Design review of the part built by this model. Coordinates are the model's own, in mm. A direction names the side the tool comes from. Coordinates: 2 decimals unless noted, no trailing zeros. Loops run counter-clockwise (first coordinate to the right, second up) from the corner with the lowest first, then second, coordinate; pieces in that order, holes last. Notation, with made-up numbers: (19, 44.25) -> (30, 44.25) arc R31 cw to (30, 73.25) -> close; hole circle Ø1 at (47.25, 49.25). An arc over 180 degrees is marked (long way). Answer in a Markdown table with one row per item.
```python
from build123d import *

# Parameters (mm, degrees)
BOSS_EXTRUDE1_DEPTH                   = 9
BOSS_EXTRUDE1_DEPTH_BACK              = 9
TAP_DRILL_FOR_M4_TAP1_D               = 3.3
TAP_DRILL_FOR_M4_TAP1_DEPTH           = 25
TAP_DRILL_FOR_M4_TAP1_TIP             = 0.991420021
TAP_DRILL_FOR_M4_TAP1_ON_FACE_2_D     = 3.3
TAP_DRILL_FOR_M4_TAP1_ON_FACE_2_DEPTH = 25
TAP_DRILL_FOR_M4_TAP1_ON_FACE_2_TIP   = 0.991420021
TAP_DRILL_FOR_M4_TAP1_ON_FACE_3_D     = 3.3
TAP_DRILL_FOR_M4_TAP1_ON_FACE_3_DEPTH = 25
TAP_DRILL_FOR_M4_TAP1_ON_FACE_3_TIP   = 0.991420021
TAP_DRILL_FOR_M4_TAP1_ON_FACE_4_D     = 3.3
TAP_DRILL_FOR_M4_TAP1_ON_FACE_4_DEPTH = 25
TAP_DRILL_FOR_M4_TAP1_ON_FACE_4_TIP   = 0.991420021
TAP_DRILL_FOR_M4_TAP1_ON_FACE_5_D     = 3.3
TAP_DRILL_FOR_M4_TAP1_ON_FACE_5_DEPTH = 25
TAP_DRILL_FOR_M4_TAP1_ON_FACE_5_TIP   = 0.991420021
FILLET2_R                             = 2


with BuildPart() as part:
    # Sketch1 → Boss-Extrude1 (new, two sides: drawn at the far end of the back side and taken through both)
    with BuildSketch(Plane.XY.offset(-BOSS_EXTRUDE1_DEPTH_BACK)):
        with BuildLine():
            Line((66.491800306, -127.729559978), (66.491800306, -83.193091613))
            ThreePointArc((66.491800306, -83.193091613), (0, -106.5), (-66.491800306, -83.193091613))
            Line((-66.491800306, -83.193091613), (-66.491800306, -127.729559978))
            ThreePointArc((-66.491800306, -127.729559978), (0, -144), (66.491800306, -127.729559978))
        make_face()
    extrude(amount=BOSS_EXTRUDE1_DEPTH + BOSS_EXTRUDE1_DEPTH_BACK)

    # Tap Drill for M4 Tap1
    with Locations(Plane(origin=(-32.025167647, -101.570855255, 0), x_dir=(0.953716950748, -0.300705799504, 0), z_dir=(0.300705799504, 0.953716950748, 0))):
        with Locations((0, 0)):
            Hole(TAP_DRILL_FOR_M4_TAP1_D / 2, depth=TAP_DRILL_FOR_M4_TAP1_DEPTH)
            with Locations((0, 0, -(TAP_DRILL_FOR_M4_TAP1_DEPTH + TAP_DRILL_FOR_M4_TAP1_TIP / 2))):  # 118° drill point
                Cone(0, TAP_DRILL_FOR_M4_TAP1_D / 2, TAP_DRILL_FOR_M4_TAP1_TIP, mode=Mode.SUBTRACT)

    # Tap Drill for M4 Tap1 on face 2
    with Locations(Plane(origin=(32.025167647, -101.570855255, 0), x_dir=(0.953716897702, 0.300705967746, 0), z_dir=(-0.300705967746, 0.953716897702, 0))):
        with Locations((0, 0)):
            Hole(TAP_DRILL_FOR_M4_TAP1_ON_FACE_2_D / 2, depth=TAP_DRILL_FOR_M4_TAP1_ON_FACE_2_DEPTH)
            with Locations((0, 0, -(TAP_DRILL_FOR_M4_TAP1_ON_FACE_2_DEPTH + TAP_DRILL_FOR_M4_TAP1_ON_FACE_2_TIP / 2))):  # 118° drill point
                Cone(0, TAP_DRILL_FOR_M4_TAP1_ON_FACE_2_D / 2, TAP_DRILL_FOR_M4_TAP1_ON_FACE_2_TIP, mode=Mode.SUBTRACT)

    # Tap Drill for M4 Tap1 on face 3
    with Locations(Plane(origin=(-55.106414261, -133.038652682, 0), x_dir=(-0.923879753837, 0.382682898036, 0), z_dir=(-0.382682898036, -0.923879753837, 0))):
        with Locations((0, 0)):
            Hole(TAP_DRILL_FOR_M4_TAP1_ON_FACE_3_D / 2, depth=TAP_DRILL_FOR_M4_TAP1_ON_FACE_3_DEPTH)
            with Locations((0, 0, -(TAP_DRILL_FOR_M4_TAP1_ON_FACE_3_DEPTH + TAP_DRILL_FOR_M4_TAP1_ON_FACE_3_TIP / 2))):  # 118° drill point
                Cone(0, TAP_DRILL_FOR_M4_TAP1_ON_FACE_3_D / 2, TAP_DRILL_FOR_M4_TAP1_ON_FACE_3_TIP, mode=Mode.SUBTRACT)

    # Tap Drill for M4 Tap1 on face 4
    with Locations(Plane(origin=(0, -144, 0), x_dir=(0, 0, -1), z_dir=(0, -1, 0))):
        with Locations((0, 0)):
            Hole(TAP_DRILL_FOR_M4_TAP1_ON_FACE_4_D / 2, depth=TAP_DRILL_FOR_M4_TAP1_ON_FACE_4_DEPTH)
            with Locations((0, 0, -(TAP_DRILL_FOR_M4_TAP1_ON_FACE_4_DEPTH + TAP_DRILL_FOR_M4_TAP1_ON_FACE_4_TIP / 2))):  # 118° drill point
                Cone(0, TAP_DRILL_FOR_M4_TAP1_ON_FACE_4_D / 2, TAP_DRILL_FOR_M4_TAP1_ON_FACE_4_TIP, mode=Mode.SUBTRACT)

    # Tap Drill for M4 Tap1 on face 5
    with Locations(Plane(origin=(55.106414261, -133.038652682, 0), x_dir=(-0.923879753837, -0.382682898036, 0), z_dir=(0.382682898036, -0.923879753837, 0))):
        with Locations((0, 0)):
            Hole(TAP_DRILL_FOR_M4_TAP1_ON_FACE_5_D / 2, depth=TAP_DRILL_FOR_M4_TAP1_ON_FACE_5_DEPTH)
            with Locations((0, 0, -(TAP_DRILL_FOR_M4_TAP1_ON_FACE_5_DEPTH + TAP_DRILL_FOR_M4_TAP1_ON_FACE_5_TIP / 2))):  # 118° drill point
                Cone(0, TAP_DRILL_FOR_M4_TAP1_ON_FACE_5_D / 2, TAP_DRILL_FOR_M4_TAP1_ON_FACE_5_TIP, mode=Mode.SUBTRACT)

    # Fillet2
    fillet2_edges = [part.edges().sort_by_distance(p)[0] for p in [
        (-66.491800306, -105.461325795, 9),
        (66.491800306, -105.461325795, 9),
        (66.491800306, -83.193091613, 0),
        (-66.491800306, -83.193091613, 0),
    ]]
    fillet(fillet2_edges, radius=FILLET2_R)


solid = part.part
```
(1) Take a section at B-B on y = -121. Count the separate pieces of the cut face and the enclosed holes in it, and give its area (3 significant figures).
Evaluation:
| item | result |
|---|---|
| separate pieces | 1 |
| enclosed holes | 5 |
| area | 2,350 mm² |
(2) Tool access review of faces 1 (the cylindrical face through (-65.36, -85.45, 0.13)), 2 (the cylindrical face through (1.115, -131.325, -1.216)), 3 (the conical face through (-44.961, -109.294, -0.013)): name each direction out of +Z, -Z, +X, -X, +Y, -Y from which nothing blocks a thin tool from reaching the whole face with its end or side.
Evaluation:
| item | result |
|---|---|
| face 1 | +Z, -Z, +Y |
| face 2 | -Y |
| face 3 | none |
(3) Take a section at A-A on z = -6.25. Give the boundary of the cut face in (x, y), and give its area (3 significant figures).
Evaluation:
| item | result |
|---|---|
| outline | (-66.49, -127.73) arc R144 ccw to (66.49, -127.73) -> (66.49, -87.25) arc R2 ccw to (63.3, -85.64) arc R106.5 cw to (-63.3, -85.64) arc R2 ccw to (-66.49, -87.25) -> close |
| area | 5,260 mm² |
(4) For pin 1 (2 mm diameter, centred on x = -33, z = -4, fed in from +Y); pin 2 (8 mm diameter, centred on x = -32.5, z = -3, fed in from -Y); pin 3 (4 mm diameter, centred on x = 39.5, z = 0, fed in from +Y); pin 4 (4 mm diameter, centred on x = 0, z = 0, fed in from -Y), all flat-tipped, find the tip position at first contact; note any pin that passes through.
Evaluation:
| item | result |
|---|---|
| pin 1 | stops at y = -100.93 |
| pin 2 | stops at y = -141.15 |
| pin 3 | stops at y = -98.08 |
| pin 4 | stops at y = -144 |
(5) To check wall thickness, follow probe 1 along Z at (x, y) = (0, -132); probe 2 along Y at (x, z) = (-0.5, -2.25); probe 3 along Y at (x, z) = (-0.5, 1). State the ranges of each line that lie inside material, in increasing order.
Evaluation:
| item | result |
|---|---|
| probe 1 | z = -9 to -1.65, 1.65 to 9 |
| probe 2 | y = -144 to -106.5 |
| probe 3 | y = -118.68 to -106.5 |
(6) Draft analysis for pull direction Y (two halves, no side actions). For faces 4 (the flat face through (66.492, -108, -1)), 5 (the cylindrical face through (48.733, -121.959, -0.073)), 6 (the cylindrical face through (0.949, -106.496, -0.126)), state which applies: pulls with the +Y half, pulls with the -Y half, needs draft (parallel to the pull), parting line crosses it, or undercut.
Evaluation:
| item | result |
|---|---|
| face 4 | needs draft |
| face 5 | undercut |
| face 6 | pulls with the +Y half |
(7) Take a section at C-C on x = -23. Give the boundary of the cut face in (y, z), and give its area (3 significant figures).
Evaluation:
| item | result |
|---|---|
| outline | (-142.15, -9) -> (-103.99, -9) -> (-103.99, 9) -> (-142.15, 9) -> close |
| area | 687 mm² |
